For this review, take the finished solid that the model builds, in its own axes (mm). A direction names the side the tool comes from. Coordinates: 2 decimals unless noted, no trailing zeros. Write each loop counter-clockwise with the first axis right and the second up, starting at its lowest first coordinate (ties: lowest second). Pieces come first, ordered by that corner, then holes. Notation, with made-up numbers: M 3.5,77.25 L 59.5,77.25 A20 cw 59.5,91.25 Z; hole C -34,44 d5. An arc over 180 degrees is marked long. One line per question, with ' | ' between items.
from build123d import *

# Parameters (mm, degrees)
F0_W      = 170
F0_H      = 210
F1_DEPTH  = 2
F2_W      = 15
F2_H      = 20
F3_DEPTH  = 2
F4_W      = 2
F4_H      = 20
F5_DEPTH  = 5
F7_DEPTH  = 2.001
F9_DEPTH  = 2.0010001
F11_DEPTH = 2.0010001
F12_W     = 2
F12_H     = 5
F13_DEPTH = 2.0010001


with BuildPart() as f1:
    # F0 (on Top) → F1 (new body)
    with BuildSketch(Plane.XY):
        with Locations((85, 105)):
            Rectangle(F0_W, F0_H)
    extrude(amount=F1_DEPTH)

    # F2 (on face) → F3 (join)
    with BuildSketch(Plane.XY.offset(2)):
        with Locations((-7.5, 105)):
            Rectangle(F2_W, F2_H)
        with Locations((177.5, 105)):
            Rectangle(F2_W, F2_H)
    extrude(amount=-F3_DEPTH)

    # F4 (on face) → F5 (join)
    with BuildSketch(Plane.XY.offset(2)):
        with Locations((184, 105)):
            Rectangle(F4_W, F4_H)
        with Locations((-14, 105)):
            Rectangle(F4_W, F4_H)
    extrude(amount=F5_DEPTH)

    # F6 (on face) → F7 (cut, through all)
    with BuildSketch(Plane.XY.offset(2)):
        with BuildLine():
            add(Edge.make_bspline(
                [(24.7591678446, 179.4151456037), (2.9330243604, 152.697989574), (0, 115)],
                knots=[3.9247129048, 3.9247129048, 3.9247129048, 4.6170063214, 4.6170063214, 4.6170063214], degree=2, weights=[1, 0.940687021, 1]))
            Line((24.7591678446, 179.4151456037), (0, 210))
            Line((0, 210), (0, 115))
        make_face()
        with BuildLine():
            add(Edge.make_bspline(
                [(85, 210), (49.7449642279, 210), (24.7591678446, 179.4151456037)],
                knots=[3.1415926536, 3.1415926536, 3.1415926536, 3.9247129048, 3.9247129048, 3.9247129048], degree=2, weights=[1, 0.9243147928, 1]))
            Line((85, 210), (0, 210))
            Line((0, 210), (24.7591678446, 179.4151456037))
        make_face()
        with BuildLine():
            add(Edge.make_bspline(
                [(145.2408321554, 179.4151456037), (120.2550357721, 210), (85, 210)],
                knots=[2.3584724024, 2.3584724024, 2.3584724024, 3.1415926536, 3.1415926536, 3.1415926536], degree=2, weights=[1, 0.9243147928, 1]))
            Line((145.2408321554, 179.4151456037), (170, 210))
            Line((170, 210), (85, 210))
        make_face()
        with BuildLine():
            add(Edge.make_bspline(
                [(170, 115), (167.0669756396, 152.697989574), (145.2408321554, 179.4151456037)],
                knots=[1.6661789858, 1.6661789858, 1.6661789858, 2.3584724024, 2.3584724024, 2.3584724024], degree=2, weights=[1, 0.940687021, 1]))
            Line((170, 115), (170, 210))
            Line((170, 210), (145.2408321554, 179.4151456037))
        make_face()
        with BuildLine():
            Line((0, 0), (24.7591678446, 30.5848543963))
            add(Edge.make_bspline(
                [(0, 95), (2.9330243604, 57.302010426), (24.7591678446, 30.5848543963)],
                knots=[4.8077716394, 4.8077716394, 4.8077716394, 5.500065056, 5.500065056, 5.500065056], degree=2, weights=[1, 0.940687021, 1]))
            Line((0, 95), (0, 0))
        make_face()
        with BuildLine():
            Line((0, 0), (85, 0))
            add(Edge.make_bspline(
                [(24.7591678446, 30.5848543963), (49.7449642279, 0), (85, 0)],
                knots=[5.500065056, 5.500065056, 5.500065056, 6.2831853072, 6.2831853072, 6.2831853072], degree=2, weights=[1, 0.9243147928, 1]))
            Line((24.7591678446, 30.5848543963), (0, 0))
        make_face()
        with BuildLine():
            Line((170, 0), (145.2408321554, 30.5848543963))
            add(Edge.make_bspline(
                [(85, 0), (120.2550357721, 0), (145.2408321554, 30.5848543963)],
                knots=[0, 0, 0, 0.7831202512, 0.7831202512, 0.7831202512], degree=2, weights=[1, 0.9243147928, 1]))
            Line((85, 0), (170, 0))
        make_face()
        with BuildLine():
            Line((170, 0), (170, 95))
            add(Edge.make_bspline(
                [(145.2408321554, 30.5848543963), (167.0669756396, 57.302010426), (170, 95)],
                knots=[0.7831202512, 0.7831202512, 0.7831202512, 1.4754136678, 1.4754136678, 1.4754136678], degree=2, weights=[1, 0.940687021, 1]))
            Line((145.2408321554, 30.5848543963), (170, 0))
        make_face()
    extrude(amount=-F7_DEPTH, mode=Mode.SUBTRACT)

    # F8 (on face) → F9 (cut, through all)
    with BuildSketch(Plane.XY.offset(2)):
        Polygon((140, 37.5), (133.8961270562, 37.5), (128.7345343242, 30.1284816281), (132.8302945456, 27.2605994464), align=None)
        Polygon((135.9042397786, 40.3678821818), (133.8961270562, 37.5), (140, 37.5), align=None)
        Polygon((140, 37.5), (140, 46.2172339781), (135.9042397786, 40.3678821818), align=None)
        Polygon((143.0739452329, 50.6072827354), (140, 46.2172339781), (140, 37.5), (147.1697054544, 47.7394005536), align=None)
        Polygon((36.1038729438, 37.5), (30, 37.5), (37.1697054544, 27.2605994464), (41.2654656758, 30.1284816281), align=None)
        Polygon((34.0957602214, 40.3678821818), (30, 37.5), (36.1038729438, 37.5), align=None)
        Polygon((34.0957602214, 40.3678821818), (30, 46.2172339781), (30, 37.5), align=None)
        Polygon((30, 37.5), (30, 46.2172339781), (26.9260547671, 50.6072827354), (22.8302945456, 47.7394005536), align=None)
    extrude(amount=-F9_DEPTH, mode=Mode.SUBTRACT)

    # F10 (on face) → F11 (cut, through all)
    with BuildSketch(Plane.XY.offset(2)):
        with BuildLine():
            Line((135.1302650927, 190), (130, 190))
            Line((130, 190), (130, 115))
            Line((130, 115), (146, 115))
            Line((146, 115), (146, 178.4740497466))
            add(Edge.make_bspline(
                [(135.1302650927, 190), (137.306371465, 188.0593608414), (139.4104340586, 186.0222842528), (141.4370654471, 183.8965010357), (143.381737679, 181.6908438843), (145.3934634846, 179.2283111754), (145.5457000719, 179.0407818641), (145.6975377618, 178.8525601554), (145.8489724333, 178.6636485868), (146, 178.4740497466)],
                knots=[2.9839924319, 2.9839924319, 2.9839924319, 2.9839924319, 2.9839924319, 2.9839924319, 3.1415926536, 3.1415926536, 3.1415926536, 3.1415926536, 3.154531604, 3.154531604, 3.154531604, 3.154531604, 3.154531604, 3.154531604], degree=5, weights=[0.999407942, 0.9995850974, 0.9997589565, 0.999907202, 1, 1, 0.9999995139, 0.9999985599, 0.9999971556, 0.9999953185]))
        make_face()
        with BuildLine():
            Line((40, 190), (34.8697349073, 190))
            add(Edge.make_bspline(
                [(24, 178.4740497466), (24.1510275667, 178.6636485868), (24.3024622382, 178.8525601554), (24.4542999281, 179.0407818641), (24.6065365154, 179.2283111754), (26.618262321, 181.6908438843), (28.5629345529, 183.8965010357), (30.5895659414, 186.0222842528), (32.693628535, 188.0593608414), (34.8697349073, 190)],
                knots=[4.6041400787, 4.6041400787, 4.6041400787, 4.6041400787, 4.6041400787, 4.6041400787, 4.6170063214, 4.6170063214, 4.6170063214, 4.6170063214, 4.773720941, 4.773720941, 4.773720941, 4.773720941, 4.773720941, 4.773720941], degree=5, weights=[0.9999953185, 0.9999971556, 0.9999985599, 0.9999995139, 1, 1, 0.999907202, 0.9997589565, 0.9995850974, 0.999407942]))
            Line((24, 178.4740497466), (24, 115))
            Line((24, 115), (40, 115))
            Line((40, 115), (40, 190))
        make_face()
        with BuildLine():
            add(Edge.make_bspline(
                [(34.8697349073, 190), (35.8666495511, 190.8890427509), (36.8786886023, 191.7578499358), (37.9053142385, 192.6056593139), (38.9459535543, 193.4317626189), (40, 194.2355073866)],
                knots=[4.773720941, 4.773720941, 4.773720941, 4.773720941, 4.773720941, 4.773720941, 4.8454962601, 4.8454962601, 4.8454962601, 4.8454962601, 4.8454962601, 4.8454962601], degree=5, weights=[0.999407942, 0.9993268048, 0.9992449761, 0.9991646, 0.9990874899, 0.9990151282]))
            Line((34.8697349073, 190), (40, 190))
            Line((40, 190), (40, 194.2355073866))
        make_face()
        with BuildLine():
            add(Edge.make_bspline(
                [(130, 194.2355073866), (131.0540464457, 193.4317626189), (132.0946857615, 192.6056593139), (133.1213113977, 191.7578499358), (134.1333504489, 190.8890427509), (135.1302650927, 190)],
                knots=[2.911811507, 2.911811507, 2.911811507, 2.911811507, 2.911811507, 2.911811507, 2.9839924319, 2.9839924319, 2.9839924319, 2.9839924319, 2.9839924319, 2.9839924319], degree=5, weights=[0.9990151282, 0.9990874899, 0.9991646, 0.9992449761, 0.9993268048, 0.999407942]))
            Line((130, 194.2355073866), (130, 190))
            Line((130, 190), (135.1302650927, 190))
        make_face()
    extrude(amount=-F11_DEPTH, mode=Mode.SUBTRACT)

    # F12 (on face) → F13 (cut, through all)
    with BuildSketch(Plane.XY.offset(2)):
        with Locations((45, 136.5)):
            Rectangle(F12_W, F12_H)
        with Locations((66, 136.5)):
            Rectangle(F12_W, F12_H)
        with Locations((104, 136.5)):
            Rectangle(F12_W, F12_H)
        with Locations((125, 136.5)):
            Rectangle(F12_W, F12_H)
    extrude(amount=-F13_DEPTH, mode=Mode.SUBTRACT)


solid = f1.part
1. Take a section at B-B on y = 106.5. State the section outline as (x, z) points.
Computed values:
outline: M -15,0 L 185,0 L 185,7 L 183,7 L 183,2 L -13,2 L -13,7 L -15,7 Z
2. Take a section at C-C on x = 173. State the section outline as (y, z) points, plus the area to 3 significant figures.
Computed values:
outline: M 95,0 L 115,0 L 115,2 L 95,2 Z | area: 40.0 mm2
3. Draft analysis for pull direction X (two halves, no side actions). For faces 4 (the flat face through (179, 115, 1)), 5 (the flat face through (29.9, 37.64, 1.01)), 6 (the flat face through (-15, 105, 4)), state which applies: pulls with the +X half, pulls with the -X half, needs draft (parallel to the pull), parting line crosses it, or undercut.
Computed values:
face 4: needs draft | face 5: undercut | face 6: pulls with the -X half
4. Clearance check with flat-ended pins moving along their axes: P1, Ø0.6, axis at x = 103.5, z = 1, coming from the +Y side; P2, Ø1, axis at x = 125, z = 1, coming from the -Y side; P3, Ø0.6, axis at y = 137.5, z = 1, coming from the +X side. State where each tip first meets the part, or that it passes through.
Computed values:
P1: stops at y = 207.59 | P2: stops at y = 11.91 | P3: stops at x = 166.27
5. Machinability: for faces 1 (the flat face through (139.9, 37.36, 1.01)), 2 (the flat face through (183, 105, 4)), 3 (the flat face through (-9, 115, 1)), which of the approach directions +Z, -Z, +X, -X, +Y, -Y give a long, thin tool a straight path to every point of the face, cutting with its end or side? Answer none if there is none.
Computed values:
face 1: +Z, -Z | face 2: +Z, +Y, -Y | face 3: +Z, -Z, -X, +Y
6. Take a section at D-D on y = 141.5. Give the number of separate pieces and of enclosed holes in the cut face, plus the area to 3 significant figures.
Computed values:
separate pieces: 3 | enclosed holes: 0 | area: 256 mm2
7. Take a section at A-A on z = 4. State the section outline as (x, y) points, plus the area to 3 significant figures.
Computed values:
outline: M -15,95 L -13,95 L -13,115 L -15,115 Z; M 183,95 L 185,95 L 185,115 L 183,115 Z | area: 80.0 mm2
8. For line 1 along X through (y, z) = (45.5, 1); line 2 along X through (y, z) = (176.5, 1); line 3 along Z through (x, y) = (111, 183.5), list the stretches that pass through material, from the lowest coordinate up.
Computed values:
line 1: x = 14.64 to 24.4, 30.5 to 139.5, 145.6 to 155.36 | line 2: x = 22.47 to 24, 40 to 130, 146 to 147.53 | line 3: z = 0 to 2
